Autodesk Inventor part; units mm, degrees
ref_plane "YZ Plane" through (0, 0, 0) normal (1, 0, 0) x (0, 1, 0)
ref_plane "XZ Plane" through (0, 0, 0) normal (0, 1, 0) x (-1, 0, 0)
ref_plane "XY Plane" through (0, 0, 0) normal (0, 0, 1) x (1, 0, 0)
ref_plane "Arbeitsebene1" through (-38.5744, -30.9423, 15.3122) normal (1, 0, 0) x (0, 1, 0)
sketch "Skizze1" plane through (-38.5744, -30.9423, 15.3122) normal (1, 0, 0) x (0, 1, 0)
  circle A0 centre (-3.7508, 1.8008) radius 1.4
  line L0 (-1.2508, 11.8008) -> (-6.2508, 11.8008)
  line L1 (-6.2508, 11.8008) -> (-6.2508, -8.1992)
  line L2 (-6.2508, -8.1992) -> (-1.2508, -8.1992)
  line L3 (-1.2508, -8.1992) -> (-1.2508, 11.8008)
  line L4 (-1.2508, 11.8008) -> (-6.2508, -8.1992) construction
  line L5 (-6.2508, 11.8008) -> (-1.2508, -8.1992) construction
  circle A1 centre (-3.7508, 1.8008) radius 1.6
  point P0 (30.9423, -15.3122)
  dimension "d0" = 5
  dimension "d1" = 20
  dimension "d4" = 0.2
extrude "Extrusion1" add sketch "Skizze1" along normal blind 2 contours L3 L2 L1 L0
sketch "Skizze2" plane through (-38.5744, -30.9423, 15.3122) normal (-1, 0, 0) x (0, 0, 1)
  circle A0 centre (1.8008, -3.7508) radius 1.6
  line L0 (11.8008, -1.2508) -> (11.8008, -6.2508)
  line L1 (11.8008, -6.2508) -> (-8.1992, -6.2508)
  line L2 (-8.1992, -6.2508) -> (-8.1992, -1.2508)
  line L3 (-8.1992, -1.2508) -> (11.8008, -1.2508)
  line L4 (-8.1992, -6.2508) -> (-8.1992, -1.2508)
  line L5 (11.8008, -6.2508) -> (-8.1992, -6.2508)
  line L6 (-8.1992, -1.2508) -> (-5.1992, -1.2508)
  line L7 (-5.1992, -1.2508) -> (-5.1992, -6.2508)
  line L8 (-5.1992, -6.2508) -> (-8.1992, -6.2508)
  line L9 (-8.1992, -6.2508) -> (-8.1992, -1.2508)
  line L10 (-8.1992, -1.2508) -> (11.8008, -1.2508)
  line L11 (11.8008, -1.2508) -> (8.8008, -1.2508)
  line L12 (8.8008, -1.2508) -> (8.8008, -6.2508)
  line L13 (8.8008, -6.2508) -> (11.8008, -6.2508)
  line L14 (11.8008, -6.2508) -> (11.8008, -1.2508)
  point P0 (-15.3122, 30.9423)
  dimension "d5" = 3
  dimension "d6" = 3
extrude "Extrusion2" add sketch "Skizze2" along normal blind 1 contours L0 L1 L12 L3 | L7 L1 L2 L3
properties part number "03_Camera_Clip"
Here's how the part is built. I have some questions about the finished solid (model axes, mm). A direction names the side the tool comes from. Coordinates: 2 decimals unless noted, no trailing zeros. Order: outer loops, then holes, each group sorted by start corner. A loop starts at its lowest first (then second) coordinate and runs counter-clockwise, first axis right, second up.
Item 1: If we section it at C-C, the plane y = -32.75: List the corners of the cut face in (x, z) for me.
Response values:
outline: (-39.57, 7.11) - (-36.57, 7.11) - (-36.57, 27.11) - (-39.57, 27.11) - (-39.57, 24.11) - (-38.57, 24.11) - (-38.57, 10.11) - (-39.57, 10.11) - close
Item 2: I need wall thicknesses on probe 1 along Z at (x, y) = (-39.15, -34.85); probe 2 along X at (y, z) = (-36.8, 20.75); probe 3 along Z at (x, y) = (-38.5, -33.35). Which ranges of each line are inside material? Lowest first, please.
Response values:
probe 1: z = 7.11 to 10.11, 24.11 to 27.11
probe 2: x = -38.57 to -36.57
probe 3: z = 7.11 to 16.24, 17.98 to 27.11
Item 3: Which directions (+Z, -Z, +X, -X, +Y, -Y) give clear straight access to the entire face, cutting with the end or side of a thin tool? Please do faces 1 (the face through (-39.574, -35, 9)), 2 (the face through (-39, -35, 24.113)).
Response values:
face 1: +Z, -Z, -X, +Y, -Y
face 2: -X, +Y, -Y
Item 4: If we section it at D-D, the plane z = 17.5: List the corners of the cut face in (x, y) for me, then the cut area to 3 significant figures.
Response values:
outline: (-38.57, -37.19) - (-36.57, -37.19) - (-36.57, -36.25) - (-38.57, -36.25) - close; (-38.57, -33.14) - (-36.57, -33.14) - (-36.57, -32.19) - (-38.57, -32.19) - close
area: 3.79 mm2
Item 5: Thinking about a two-plate mould opening in Y: for faces 3 (the face through (-38, -32.193, 17)), 4 (the face through (-37.588, -35.04, 18.675)), 5 (the face through (-38, -37.193, 17)), which applies, pulls with the +Y half, pulls with the -Y half, needs draft (parallel to the pull), parting line crosses it, or undercut?
Response values:
face 3: pulls with the +Y half
face 4: undercut
face 5: pulls with the -Y half
Item 6: I'm going to push a flat-ended pin straight in: pin 1 Ø1.9 at (y, z) = (-34.69, 17.11) entering from +X. Where does the tip first touch, or does it pass through?
Response values:
pin 1: passes through
Item 7: If we section it at B-B, the plane y = -34: List the corners of the cut face in (x, z) for me, then the cut area to 3 significant figures.
Response values:
outline: (-39.57, 7.11) - (-36.57, 7.11) - (-36.57, 15.67) - (-38.57, 15.67) - (-38.57, 10.11) - (-39.57, 10.11) - close; (-39.57, 24.11) - (-38.57, 24.11) - (-38.57, 18.56) - (-36.57, 18.56) - (-36.57, 27.11) - (-39.57, 27.11) - close
area: 40.2 mm2
Item 8: If we section it at A-A, the plane x = -39.1: List the corners of the cut face in (y, z) for me.
Response values:
outline: (-37.19, 7.11) - (-32.19, 7.11) - (-32.19, 10.11) - (-37.19, 10.11) - close; (-37.19, 24.11) - (-32.19, 24.11) - (-32.19, 27.11) - (-37.19, 27.11) - close
